Here's how the part is built. I have some questions about the finished solid (model axes, mm). Face numbers are marked on the shaded views. A direction names the side the tool comes from. Coordinates: 2 decimals unless noted, no trailing zeros. Loops run counter-clockwise (first coordinate to the right, second up) from the corner with the lowest first, then second, coordinate; pieces in that order, holes last.
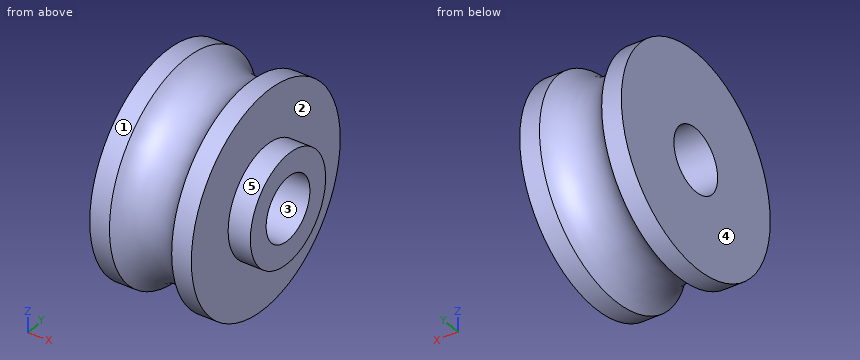
```python
from build123d import *


with BuildPart() as f2:
    # F0 (on Top) → F2 (revolve)
    with BuildSketch(Plane.XY):
        with BuildLine():
            Line((0, 6), (0, 0))
            Line((0, 0), (1.549061, 0))
            ThreePointArc((1.549061, 0), (4, 1.27), (6.450939, 0))
            Line((6.450939, 0), (8, 0))
            Line((8, 0), (8, 4.2))
            Line((8, 4.2), (9.75, 4.2))
            Line((9.75, 4.2), (9.75, 6))
            Line((9.75, 6), (0, 6))
        make_face()
    revolve(axis=Axis((10.455161, 8.5, 0), (1, 0, 0)))


solid = f2.part
```
1. I want a section at B-B (z = 0). Please give me the cut outline in (x, y).
2. I want a section at C-C (x = 0.5). Please give me the cut outline in (y, z), then the cut area to 3 significant figures.
3. I want a section at A-A (y = 8.5). Please give me the cut outline in (x, z), then the cut area to 3 significant figures.
4. For pin 1 (3 mm diameter, centred on x = 7, z = 5, fed in from -Y); pin 2 (2 mm diameter, centred on x = 1.5, y = 4, fed in from +Z); pin 3 (4 mm diameter, centred on x = 6.5, z = -4.5, fed in from -Y); pin 4 (2 mm diameter, centred on y = 7.5, z = -1.5, fed in from -X), each with a flat end and sliding along its axis, tell me the tip position at first contact or that it passes through.
5. On a 3-axis mill with a long thin cutter (end or side, diameter ignored), from which of +Z, -Z, +X, -X, +Y, -Y can I reach the whole of each face in a straight line? I mean the marked faces 1 and 2. Say none if no direction works.
6. We'd pull the mould along Y, two halves only. Please class the marked faces 3, 4 and 5: +Y half, -Y half, draft (parallel to the pull), parting line (faces both ways), or undercut.
7. I want a section at D-D (x = 8.5). Please give me the cut outline in (y, z).
8. I need wall thicknesses on line 1 along Z through (x, y) = (6.5, 8.5); line 2 along Y through (x, z) = (7.25, 0); line 3 along X through (y, z) = (3, 3). Which ranges of each line are inside material? Lowest first, please.
Response values:
1. outline: (0, 0) - (1.55, 0) arc R3 cw to (6.45, 0) - (8, 0) - (8, 4.2) - (9.75, 4.2) - (9.75, 6) - (0, 6) - close; (0, 11) - (9.75, 11) - (9.75, 12.8) - (8, 12.8) - (8, 17) - (6.45, 17) arc R3 cw to (1.55, 17) - (0, 17) - close
2. outline: circle Ø17 at (8.5, 0); hole circle Ø5 at (8.5, 0)
2. area: 207 mm2
3. outline: (0, -8.5) - (1.55, -8.5) arc R3 cw to (6.45, -8.5) - (8, -8.5) - (8, -4.3) - (9.75, -4.3) - (9.75, -2.5) - (0, -2.5) - close; (0, 2.5) - (9.75, 2.5) - (9.75, 4.3) - (8, 4.3) - (8, 8.5) - (6.45, 8.5) arc R3 cw to (1.55, 8.5) - (0, 8.5) - close
3. area: 93.6 mm2
4. pin 1: stops at y = 0.75
4. pin 2: stops at z = 7.75
4. pin 3: stops at y = 0.38
4. pin 4: stops at x = 0
5. face 1: +X, -X
5. face 2: +X
6. face 3: undercut
6. face 4: draft
6. face 5: parting line
7. outline: circle Ø8.6 at (8.5, 0); hole circle Ø5 at (8.5, 0)
8. line 1: z = -8.5 to -2.5, 2.5 to 8.5
8. line 2: y = 0 to 6, 11 to 17
8. line 3: x = 0 to 8
